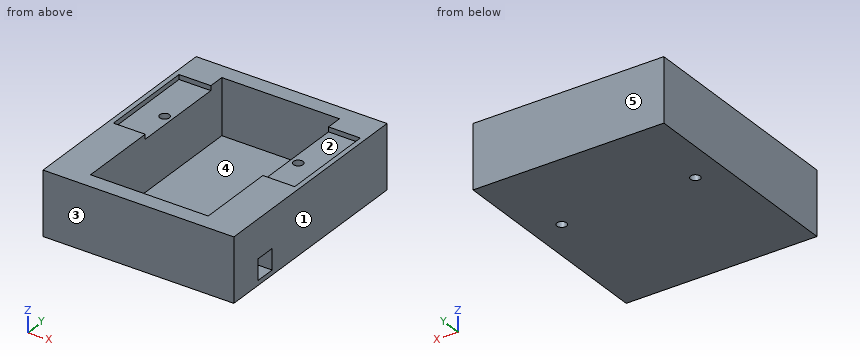
from build123d import *

# Parameters (mm, degrees)
SKETCH2_W           = 120
SKETCH2_H           = 140
BOSS_EXTRUDE1_DEPTH = 40
SKETCH3_W           = 74
SKETCH3_H           = 120
CUT_EXTRUDE1_DEPTH  = 35
SKETCH4_R           = 3
CUT_EXTRUDE2_DEPTH  = 40
SKETCH5_W           = 13
SKETCH5_H           = 13
CUT_EXTRUDE3_DEPTH  = 22
SKETCH6_W           = 20
SKETCH6_H           = 60
CUT_EXTRUDE4_DEPTH  = 3


with BuildPart() as part:
    # Sketch2 → Boss-Extrude1 (new body)
    with BuildSketch(Plane.XY):
        with Locations((-60, -70)):
            Rectangle(SKETCH2_W, SKETCH2_H)
    extrude(amount=BOSS_EXTRUDE1_DEPTH)

    # Sketch3 → Cut-Extrude1 (cut)
    with BuildSketch(Plane.XY.offset(40)):
        with Locations((-60, -70)):
            Rectangle(SKETCH3_W, SKETCH3_H)
    extrude(amount=-CUT_EXTRUDE1_DEPTH, mode=Mode.SUBTRACT)

    # Sketch4 → Cut-Extrude2 (cut)
    with BuildSketch(Plane.XY.offset(40)):
        with Locations((-102, -55)):
            Circle(SKETCH4_R)
        with Locations((-18, -55)):
            Circle(SKETCH4_R)
    extrude(amount=-CUT_EXTRUDE2_DEPTH, mode=Mode.SUBTRACT)

    # Sketch5 → Cut-Extrude3 (cut)
    with BuildSketch(Plane(origin=(0, 0, 0), x_dir=(0, 0, -1), z_dir=(1, 0, 0))):
        with Locations((-9.5, -111.5)):
            Rectangle(SKETCH5_W, SKETCH5_H)
    extrude(amount=-CUT_EXTRUDE3_DEPTH, mode=Mode.SUBTRACT)

    # Sketch6 → Cut-Extrude4 (cut)
    with BuildSketch(Plane.XY.offset(40)):
        with Locations((-107, -50)):
            Rectangle(SKETCH6_W, SKETCH6_H)
        with Locations((-13, -50)):
            Rectangle(SKETCH6_W, SKETCH6_H)
    extrude(amount=-CUT_EXTRUDE4_DEPTH, mode=Mode.SUBTRACT)


solid = part.part
The model under review builds one solid part; all positions refer to its coordinate system, in mm. Face numbers are marked on the shaded views. A direction names the side the tool comes from. Give positions to 0.01 mm unless a question says otherwise; leave off trailing zeros. Order: outer loops, then holes, each group sorted by start corner. A loop starts at its lowest first (then second) coordinate and runs counter-clockwise, first axis right, second up. Notation, with made-up numbers: M 32,8 L 84,8 A20 cw 84,33 Z; hole C 26.25,85.25 d11. An arc over 180 degrees is marked long. Use one line per item in the form item = value. Start each with the question number.
Item 1: Insertion check: pin 1 Ø14.5 at (x, y) = (-15.5, -114.5) entering from -Z; pin 2 Ø3.5 at (x, y) = (-102, -55) entering from -Z; pin 3 Ø2 at (x, y) = (-87.5, -55.5) entering from +Z; pin 4 Ø6 at (x, y) = (-12, -63.5) entering from +Z. Each pin has a flat end and moves straight along its axis. Give the tip position at first contact, or say it passes through.
Item 2: We need section C-C on z = 32. Give the boundary of the cut face in (x, y), plus the area to 3 significant figures.
Item 3: To check wall thickness, follow line 1 along Y through (x, z) = (-81, 20); line 2 along X through (y, z) = (-106, 14.5); line 3 along Z through (x, y) = (-13.5, -110.5). State the ranges of each line that lie inside material, in increasing order. Write a range as from..to.
Item 4: For the marked faces 4 and 5, list the 3-axis set-ups (+Z, -Z, +X, -X, +Y, -Y) from which the entire face can be reached by the end or side of a thin tool; tool diameter is ignored.
Item 5: The part is to be moulded in two halves that separate along X. For the marked faces 1, 2 and 3, say which applies: pulls with the +X half, pulls with the -X half, needs draft (parallel to the pull), parting line crosses it, or undercut.
Item 6: We need section A-A on x = -18. Give the boundary of the cut face in (y, z).
Item 7: We need section D-D on x = -102. Give the boundary of the cut face in (y, z).
Item 8: We need section B-B on y = -55. Give the boundary of the cut face in (x, z), plus the area to 3 significant figures.
Completed:
q1.pin_1 = 0
q1.pin_2 = through
q1.pin_3 = 5
q1.pin_4 = 37
q2.outline = M -120,-140 L 0,-140 L 0,0 L -120,0 Z; hole C -102,-55 d6; hole M -97,-130 L -23,-130 L -23,-10 L -97,-10 Z; hole C -18,-55 d6
q2.area = 7,860 mm²
q3.line_1 = -140..-130, -10..0
q3.line_2 = -120..-97, -23..-22
q3.line_3 = 0..3, 16..40
q4.face_4 = +Z
q4.face_5 = +Z, -Z, +X, -X, +Y
q5.face_1 = pulls with the +X half
q5.face_2 = undercut
q5.face_3 = needs draft
q6.outline = M -140,0 L -58,0 L -58,37 L -80,37 L -80,40 L -140,40 Z; M -52,0 L 0,0 L 0,40 L -20,40 L -20,37 L -52,37 Z; hole M -118,3 L -105,3 L -105,16 L -118,16 Z
q7.outline = M -140,0 L -58,0 L -58,37 L -80,37 L -80,40 L -140,40 Z; M -52,0 L 0,0 L 0,40 L -20,40 L -20,37 L -52,37 Z
q8.outline = M -120,0 L -105,0 L -105,37 L -117,37 L -117,40 L -120,40 Z; M -99,0 L -21,0 L -21,37 L -23,37 L -23,5 L -97,5 L -97,37 L -99,37 Z; M -15,0 L 0,0 L 0,40 L -3,40 L -3,37 L -15,37 Z
q8.area = 1,650 mm²
